from build123d import *

# Parameters (mm, degrees)
F0_W      = 85.8696545474
F0_H      = 63.5460242629
F1_DEPTH  = 12.7
F2_W      = 92.7285123616
F2_H      = 86.2638354301
F3_DEPTH  = 25.4
F4_W      = 18.4039166197
F4_H      = 86.2638354301
F5_DEPTH  = 125.7651254213
F7_DEPTH  = 125.7651254213
F8_W      = 11.9450474158
F8_H      = 21.8296758831
F9_DEPTH  = 12.701
F11_DEPTH = 25.401


with BuildPart() as f1:
    # F0 (on Top) → F1 (new body)
    with BuildSketch(Plane.XY):
        with BuildLine():
            Line((-80.6561261415, -63.5460242629), (-80.6561261415, -69.8450654745))
            ThreePointArc((-80.6561261415, -69.8450654745), (-35.2602329122, -100.2452354213), (5.2135284059, -63.5460242629))
            Line((5.2135284059, -63.5460242629), (-80.6561261415, -63.5460242629))
        make_face()
        with Locations((-37.7212988678, -31.7730121315)):
            Rectangle(F0_W, F0_H)
    extrude(amount=F1_DEPTH)

    # F2 (on face) → F3 (join)
    with BuildSketch(Plane(origin=(0, 0, 0), x_dir=(-1, 0, 0), z_dir=(0, 1, 0))):
        with Locations((34.2918699607, 43.1319177151)):
            Rectangle(F2_W, F2_H)
    extrude(amount=F3_DEPTH)

    # F4 (on face) → F5 (cut, through all)
    with BuildSketch(Plane(origin=(0, 25.4, 0), x_dir=(-1, 0, 0), z_dir=(0, 1, 0))):
        with Locations((-2.8704279102, 43.1319177151)):
            Rectangle(F4_W, F4_H)
    extrude(amount=-F5_DEPTH, mode=Mode.SUBTRACT)

    # F6 (on face) → F7 (cut, through all)
    with BuildSketch(Plane(origin=(0, 25.4, 0), x_dir=(-1, 0, 0), z_dir=(0, 1, 0))):
        with BuildLine():
            Line((35.4592986405, 86.2638354301), (35.4592986405, 43.8016988337))
            ThreePointArc((35.4592986405, 43.8016988337), (42.9720902866, 36.2405068141), (50.22874102, 44.0478548408))
            Line((50.22874102, 44.0478548408), (49.4902729988, 86.2638354301))
            Line((49.4902729988, 86.2638354301), (35.4592986405, 86.2638354301))
        make_face()
        Polygon((49.4902729988, 86.2638354301), (50.22874102, 44.0478548408), (50.22874102, 86.2638354301), align=None)
    extrude(amount=-F7_DEPTH, mode=Mode.SUBTRACT)

    # F8 (on face) → F9 (cut, through all)
    with BuildSketch(Plane.XY.offset(12.7)):
        with Locations((-12.3040541075, -10.9148379415)):
            Rectangle(F8_W, F8_H)
    extrude(amount=-F9_DEPTH, mode=Mode.SUBTRACT)

    # F10 (on face) → F11 (cut, through all)
    with BuildSketch(Plane.XZ):
        Polygon((-18.2765778154, 31.0841165483), (-18.2765778154, 12.7), (-18.2765778154, 0), (-6.3315303996, 0), (-6.3315303996, 31.0841165483), align=None)
    extrude(amount=-F11_DEPTH, mode=Mode.SUBTRACT)


solid = f1.part
Here's how the part is built. I have some questions about the finished solid (model axes, mm). A direction names the side the tool comes from. Round coordinates to 2 decimals unless told otherwise and drop trailing zeros. Loops run counter-clockwise (first coordinate to the right, second up) from the corner with the lowest first, then second, coordinate; pieces in that order, holes last. Notation, with made-up numbers: (54, 48.5) -> (74, 48.5) arc R25 cw to (74, 84.5) -> close; hole circle Ø9 at (67.5, 2). An arc over 180 degrees is marked (long way). Write each question's results on one line, items separated by ' | '.
(1) If we section it at C-C, the plane x = -40: List the corners of the cut face in (y, z) for me, then the cut area to 3 significant figures.
Worked answers:
outline: (-100.34, 0) -> (25.4, 0) -> (25.4, 36.81) -> (0, 36.81) -> (0, 12.7) -> (-100.34, 12.7) -> close | area: 2,210 mm2
(2) For P1, Ø6, axis at x = -13, y = 11, coming from the -Z side; P2, Ø6, axis at x = -11.5, z = 5, coming from the +Y side; P3, Ø22.5, axis at x = -48.5, y = -66, coming from the +Z side, each with a flat end and sliding along its axis, tell me the tip position at first contact or that it passes through.
Worked answers:
P1: z = 31.08 | P2: y = -21.83 | P3: z = 12.7
(3) For faces 5 (the face through (-12, -21.83, 6)), 6 (the face through (-35.459, 13, 65)), 7 (the face through (-18.277, 7, 12)), 8 (the face through (-12, 13, 31.084)), which set-ups out of +Z, -Z, +X, -X, +Y, -Y let a thin tool reach every point of the face, with its end or its side?
Worked answers:
face 5: +Z, -Z, +X, +Y | face 6: +Z, +Y, -Y | face 7: -Z, +X, +Y | face 8: -Z, +X, +Y, -Y
(4) If we section it at D-D, the plane z = 6: List the corners of the cut face in (x, y) for me.
Worked answers:
outline: (-80.66, -69.85) arc R44.37 ccw to (-6.33, -86.55) -> (-6.33, -21.83) -> (-18.28, -21.83) -> (-18.28, 25.4) -> (-80.66, 25.4) -> close
(5) If I drill on L1, parallel to Z at x = -71, y = -71.5; L2, parallel to Y at x = -70.5, z = 59; L3, parallel to Z at x = -16, y = 10.5, over which ranges is the centre line in solid material (lowest first)?
Worked answers:
L1: 0 to 12.7 | L2: 0 to 25.4 | L3: 31.08 to 86.26
(6) If we section it at A-A, the plane z = 46.5: List the corners of the cut face in (x, y) for me.
Worked answers:
outline: (-80.66, 0) -> (-50.23, 0) -> (-50.23, 25.4) -> (-80.66, 25.4) -> close; (-35.46, 0) -> (-6.33, 0) -> (-6.33, 25.4) -> (-35.46, 25.4) -> close
(7) If we section it at B-B, the plane y = 12: List the corners of the cut face in (x, z) for me.
Worked answers:
outline: (-80.66, 0) -> (-18.28, 0) -> (-18.28, 31.08) -> (-6.33, 31.08) -> (-6.33, 86.26) -> (-35.46, 86.26) -> (-35.46, 43.8) arc R7.39 cw (long way) to (-50.23, 44.05) -> (-50.23, 86.26) -> (-80.66, 86.26) -> close
(8) We'd pull the mould along X, two halves only. Please class faces 1 (the face through (-80.656, 2, 33)), 2 (the face through (-42.81, 12.88, 36.24)), 3 (the face through (-44, -49, 12.7)), 4 (the face through (-50.229, 13, 65)): released by +X, released by -X, zero draft, split by the parting line, or undercut.
Worked answers:
face 1: released by -X | face 2: undercut | face 3: zero draft | face 4: undercut
